The listing builds one solid part. Answer for the finished solid, in the listing's coordinates (mm). A direction names the side the tool comes from. Give positions to 0.01 mm unless a question says otherwise; leave off trailing zeros. Write each loop counter-clockwise with the first axis right and the second up, starting at its lowest first coordinate (ties: lowest second). Pieces come first, ordered by that corner, then holes. Notation, with made-up numbers: (20.25, -8.5) - (57.25, -8.5) arc R19 ccw to (57.25, -0.5) - close; hole circle Ø6 at (28.25, 0). An arc over 180 degrees is marked (long way). Answer as CSV lines item,"result". Start each with the question number.
(1) For faces 1 (the face through (9.02, -13.88, 0.99)), 2 (the face through (4.108, -13.217, 2.764)), 3 (the face through (-1.678, -2.223, 2.764)), 4 (the face through (-13.36, 2.38, 0.99)), 5 (the face through (2.699, -16.624, 2.764)), determine the directions among +Z, -Z, +X, -X, +Y, -Y from which every point of the face is accessible in a straight line to the end or side of a thin tool.
(2) Find section D-D (x = -26). Write down the section's boundary in (y, z).
(3) Find section B-B (y = -1.5). Write down the section's boundary in (x, z), then the cut area to 3 significant figures.
(4) Straight lines are drawn through the part: probe 1 along Z at (x, y) = (-6, -6.5); probe 2 along X at (y, z) = (3, 1.95); probe 3 along X at (y, z) = (-9.5, 0.4). For each, find the intervals that lie inside material, in ascending order.
(5) Find section A-A (z = 1.15). Write down the section's boundary in (x, y), then the cut area to 3 significant figures.
(6) Each of these flat-tipped pins is pushed along its axis until it touches: pin 1 Ø1.6 at (x, z) = (-21, 0.5) entering from -Y; pin 2 Ø12 at (x, y) = (7.5, -26) entering from -Z; pin 3 Ø10 at (x, y) = (3.5, -10) entering from +Z. Where does it stop, or does it pass through?
(7) Find section C-C (x = 5). Write down the section's boundary in (y, z).
(8) For a pull along Y with two mould halves and no side action, classify faces 6 (the face through (-13.921, -4.329, 2.764)), 7 (the face through (0.47, 2.242, 0.986)), 8 (the face through (8, -18.975, 1)) as pulls with the +Y half, pulls with the -Y half, needs draft (parallel to the pull), parting line crosses it, or undercut.
from build123d import *

# Parameters (mm, degrees)
SALIENTE_EXTRUIR1_DEPTH = 2
SALIENTE_EXTRUIR2_DEPTH = 2
SALIENTE_EXTRUIR2_DRAFT = 72


with BuildPart() as part:
    # Croquis1 → Saliente-Extruir1 (new body)
    with BuildSketch(Plane.XY):
        Polygon((-6.350280368, -35.236671251), (-11.634129822, -18.974654774), (-28.733025837, -18.974654774), (-14.899728375, -8.924175866), (-20.183577829, 7.337840611), (-6.350280368, -2.712638297), (7.483017094, 7.337840611), (2.19916764, -8.924175866), (16.032465101, -18.974654774), (-1.066430914, -18.974654774), align=None)
    extrude(amount=SALIENTE_EXTRUIR1_DEPTH)


with BuildPart() as saliente_extruir2_tool:
    # Croquis2 → Saliente-Extruir2 (with draft: the straight prism first)
    with BuildSketch(Plane.XY.offset(2)):
        Polygon((-14.899728375, -8.924175866), (-28.733025837, -18.974654774), (-11.634129822, -18.974654774), (-6.350280368, -35.236671251), (-1.066430914, -18.974654774), (16.032465101, -18.974654774), (2.19916764, -8.924175866), (7.483017094, 7.337840611), (-6.350280368, -2.712638297), (-20.183577829, 7.337840611), align=None)
    extrude(amount=SALIENTE_EXTRUIR2_DEPTH)
    # Saliente-Extruir2: the draft: its side faces are tilted about the plane it starts from
    saliente_extruir2_sides = [saliente_extruir2_tool.faces().sort_by_distance(p)[0] for p in [
        (-17.541653102, -0.793167627, 3),
        (-21.816377106, -13.94941532, 3),
        (-20.183577829, -18.974654774, 3),
        (-8.992205095, -27.105663013, 3),
        (-3.708355641, -27.105663013, 3),
        (7.483017094, -18.974654774, 3),
        (9.115816371, -13.94941532, 3),
        (4.841092367, -0.793167627, 3),
        (0.566368363, 2.312601157, 3),
        (-13.266929099, 2.312601157, 3),
    ]]
    draft(saliente_extruir2_sides, Plane.XY.offset(2), SALIENTE_EXTRUIR2_DRAFT)


with BuildPart() as part_1:
    add(part.part)

    # Saliente-Extruir2: add saliente_extruir2_tool
    add(saliente_extruir2_tool.part)


solid = part_1.part
Result set:
1,face 1,"+Z, -Z, +X"
1,face 2,"+Z, +X"
1,face 3,"+Z, +Y"
1,face 4,"+Z, -Z, +Y"
1,face 5,"+Z, +X, -Y"
2,outline,"(-18.97, 0) - (-16.99, 0) - (-16.99, 2) - (-18.09, 2.29) - (-18.97, 2) - close"
3,outline,"(-17.31, 0) - (-8.02, 0) - (-8.02, 2) - (-13.76, 3.1) - (-17.31, 2) - close; (-4.68, 0) - (4.61, 0) - (4.61, 2) - (1.06, 3.1) - (-4.68, 2) - close"
3,area,"47.4 mm^2"
4,probe 1,"0 to 3.06"
4,probe 2,"-18.77 to -14.21, 1.51 to 6.07"
4,probe 3,"-15.69 to 2.99"
5,outline,"(-28.73, -18.97) - (-11.63, -18.97) - (-6.35, -35.24) - (-1.07, -18.97) - (16.03, -18.97) - (2.2, -8.92) - (7.48, 7.34) - (-6.35, -2.71) - (-20.18, 7.34) - (-14.9, -8.92) - close"
5,area,"622 mm^2"
6,pin 1,"y = -18.97"
6,pin 2,"through"
6,pin 3,"z = 3.66"
7,outline,"(-18.97, 0) - (-10.96, 0) - (-10.96, 2) - (-15.39, 3.16) - (-18.97, 2) - close; (-0.3, 0) - (5.53, 0) - (5.53, 2) - (3.92, 2.42) - (-0.3, 2) - close"
8,face 6,"undercut"
8,face 7,"pulls with the +Y half"
8,face 8,"pulls with the -Y half"
